Could you check a few things on this model? Use its own coordinates, in mm. A direction names the side the tool comes from. Give positions to 0.01 mm unless a question says otherwise; leave off trailing zeros. Write each loop counter-clockwise with the first axis right and the second up, starting at its lowest first coordinate (ties: lowest second). Pieces come first, ordered by that corner, then holes. Notation, with made-up numbers: (49, 83) - (71, 83) arc R22 ccw to (71, 97) - close; hole circle Ø11 at (28, -38.5). An arc over 180 degrees is marked (long way). Write item = value, one per line.
Autodesk Fusion 360 part; units mm, degrees
sketch "Esboço1" plane through (0, 0, 0) normal (0, 0, 1) x (1, 0, 0)
  line L0 (1.9999, 62) -> (2, 62)
  line L1 (15, 42) -> (21, 42)
  line L2 (15, 54) -> (15, 42)
  line L3 (2, 6) -> (2, 62)
  line L4 (1.9999, 62) -> (21, 62)
  line L5 (2, 6) -> (21, 6)
  line L6 (21, 62) -> (21, 54)
  line L7 (21, 54) -> (15, 54)
  line L8 (21, 14) -> (21, 6)
  line L9 (21, 42) -> (21, 36)
  arc A0 (21, 36) -> (21, 14) centre (21, 25) ccw
  dimension "d2" = 12
  dimension "d3" = 6
  dimension "d5" = 8
  dimension "d8" = 6
  dimension "d10" = 8
  dimension "d36" = 19
  dimension "d12" = 6
  dimension "d13" = 11
extrude "Extrusão1" add sketch "Esboço1" along normal blind 30
hole "Furo1" at (2, 47.5, 15) direction (1, 0, 0) diameter 4 depth 21 tip angle 180
hole "Furo2" at (2, 10.5, 15) direction (1, 0, 0) diameter 4 depth 21 tip angle 180
fillet "Arredondamento1" radius 1.5 8 edges at (11.5, 62, 30) (2, 62, 15) (2, 34, 30) (2, 6, 15) (11.5, 6, 30) (11.5, 6, 0) (2, 34, 0) (11.5, 62, 0)
1. Which directions (+Z, -Z, +X, -X, +Y, -Y) give clear straight access to the entire face, cutting with the end or side of a thin tool? Please do faces 4 (the face through (12.37, 6.45, 29.57)), 5 (the face through (18, 54, 15)).
Filled sheet:
face_4 = +Z, +X, -X, -Y
face_5 = +Z, -Z, +X
2. If we section it at B-B, the plane z = 22.25: Please give me the cut outline in (x, y), and give its area (3 significant figures).
Filled sheet:
outline = (2, 7.5) arc R1.5 ccw to (3.5, 6) - (21, 6) - (21, 14) arc R11 cw to (21, 36) - (21, 42) - (15, 42) - (15, 54) - (21, 54) - (21, 62) - (3.5, 62) arc R1.5 ccw to (2, 60.5) - close
area = 801 mm2
3. I need wall thicknesses on line 1 (Y direction, x = 5.5, z = 15); line 2 (Y direction, x = 13, z = 15); line 3 (Y direction, x = 16.25, z = 19.75). Which ranges of each line are inside material? Lowest first, please.
Filled sheet:
line_1 = 6 to 8.5, 12.5 to 45.5, 49.5 to 62
line_2 = 6 to 8.5, 12.5 to 17.45, 32.55 to 45.5, 49.5 to 62
line_3 = 6 to 15.08, 34.92 to 42, 54 to 62
4. If we section it at C-C, the plane x = 6: Please give me the cut outline in (y, z).
Filled sheet:
outline = (6, 1.5) arc R1.5 ccw to (7.5, 0) - (60.5, 0) arc R1.5 ccw to (62, 1.5) - (62, 28.5) arc R1.5 ccw to (60.5, 30) - (7.5, 30) arc R1.5 ccw to (6, 28.5) - close; hole circle Ø4 at (10.5, 15); hole circle Ø4 at (47.5, 15)
5. Thinking about a two-plate mould opening in Y: for faces 1 (the face through (18, 42, 15)), 2 (the face through (10, 34, 30)), 3 (the face through (2.43, 6.45, 15.19)), which applies, pulls with the +Y half, pulls with the -Y half, needs draft (parallel to the pull), parting line crosses it, or undercut?
Filled sheet:
face_1 = undercut
face_2 = needs draft
face_3 = pulls with the -Y half
6. If we section it at A-A, the plane x = 12.5: Please give me the cut outline in (y, z).
Filled sheet:
outline = (6, 1.5) arc R1.5 ccw to (7.5, 0) - (18.02, 0) - (18.02, 30) - (7.5, 30) arc R1.5 ccw to (6, 28.5) - close; (31.98, 0) - (60.5, 0) arc R1.5 ccw to (62, 1.5) - (62, 28.5) arc R1.5 ccw to (60.5, 30) - (31.98, 30) - close; hole circle Ø4 at (10.5, 15); hole circle Ø4 at (47.5, 15)
7. For pin 1 (3 mm diameter, centred on y = 10.5, z = 15, fed in from -X); pin 2 (6 mm diameter, centred on y = 49.5, z = 9.5, fed in from +X), each with a flat end and sliding along its axis, tell me the tip position at first contact or that it passes through.
Filled sheet:
pin_1 = through
pin_2 = 15
